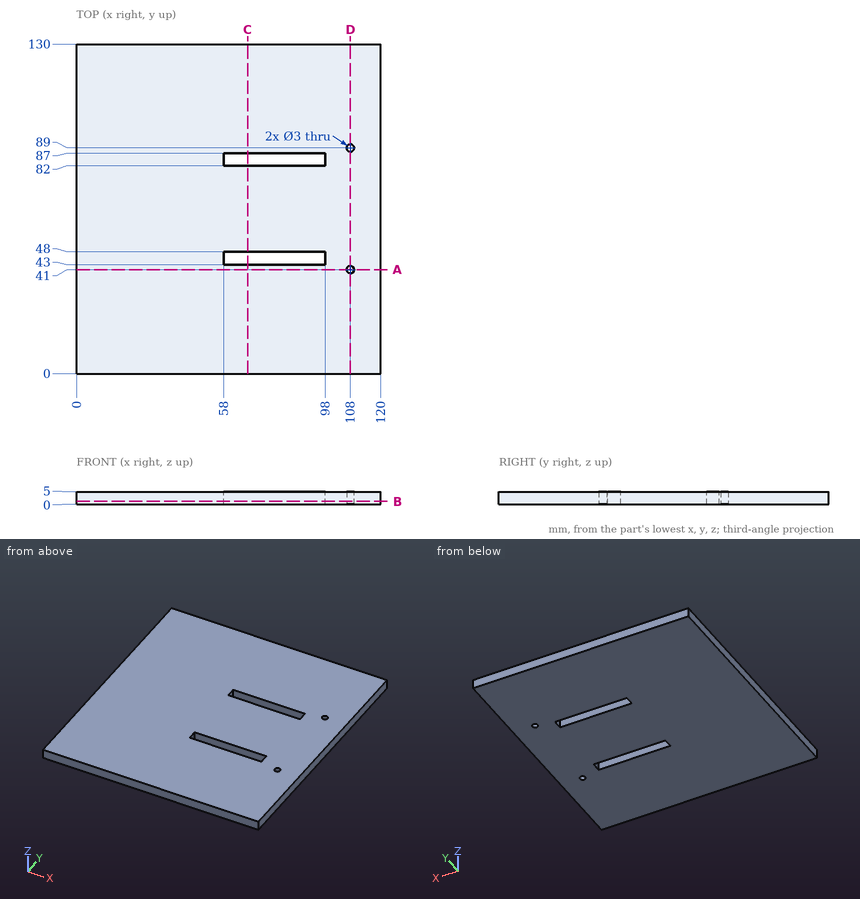
Source: three-view drawing plus pictorial views. Frame: mm from the lowest corner of the part. Coordinates: 2 decimals unless noted, no trailing zeros. Loops run counter-clockwise (first coordinate to the right, second up) from the corner with the lowest first, then second, coordinate; pieces in that order, holes last. Notation, with made-up numbers: (-36, -3) - (-3, -3) arc R21 cw to (-3, 18) - close; hole circle Ø4 at (-21, 74.25). An arc over 180 degrees is marked (long way). One line per item, written item: value. Start each with the question number.
1. Ray query, L1, parallel to Y at x = 108, z = 2.15; L2, parallel to Y at x = 87, z = 0.8; L3, parallel to X at y = 89, z = 1.4. Return the intervals inside material, ascending.
2. Section B-B (z = 1.15). Return the cut outline in (x, y).
3. Section C-C (x = 67.5). Return the cut outline in (y, z).
4. Section A-A (y = 41). Return the cut outline in (x, z).
5. Section D-D (x = 108). Return the cut outline in (y, z).
6. Contact query for a flat-ended pin moving along its axis: P1, Ø1.5, axis at y = 44.5, z = 3, coming from the -X side. Output: stop coordinate, or through.
Verdict:
1. L1: y = 0 to 39.5, 42.5 to 87.5, 90.5 to 130
1. L2: y = 0 to 43, 48 to 82, 87 to 130
1. L3: x = 0 to 106.5, 109.5 to 120
2. outline: (0, 0) - (120, 0) - (120, 130) - (0, 130) - close; hole (58, 43) - (98, 43) - (98, 48) - (58, 48) - close; hole (58, 82) - (98, 82) - (98, 87) - (58, 87) - close; hole circle Ø3 at (108, 41); hole circle Ø3 at (108, 89)
3. outline: (0, 0) - (43, 0) - (43, 5) - (0, 5) - close; (48, 0) - (82, 0) - (82, 5) - (48, 5) - close; (87, 0) - (130, 0) - (130, 5) - (87, 5) - close
4. outline: (0, 0) - (106.5, 0) - (106.5, 5) - (0, 5) - close; (109.5, 0) - (120, 0) - (120, 5) - (109.5, 5) - close
5. outline: (0, 0) - (39.5, 0) - (39.5, 5) - (0, 5) - close; (42.5, 0) - (87.5, 0) - (87.5, 5) - (42.5, 5) - close; (90.5, 0) - (130, 0) - (130, 5) - (90.5, 5) - close
6. P1: stops at x = 0
